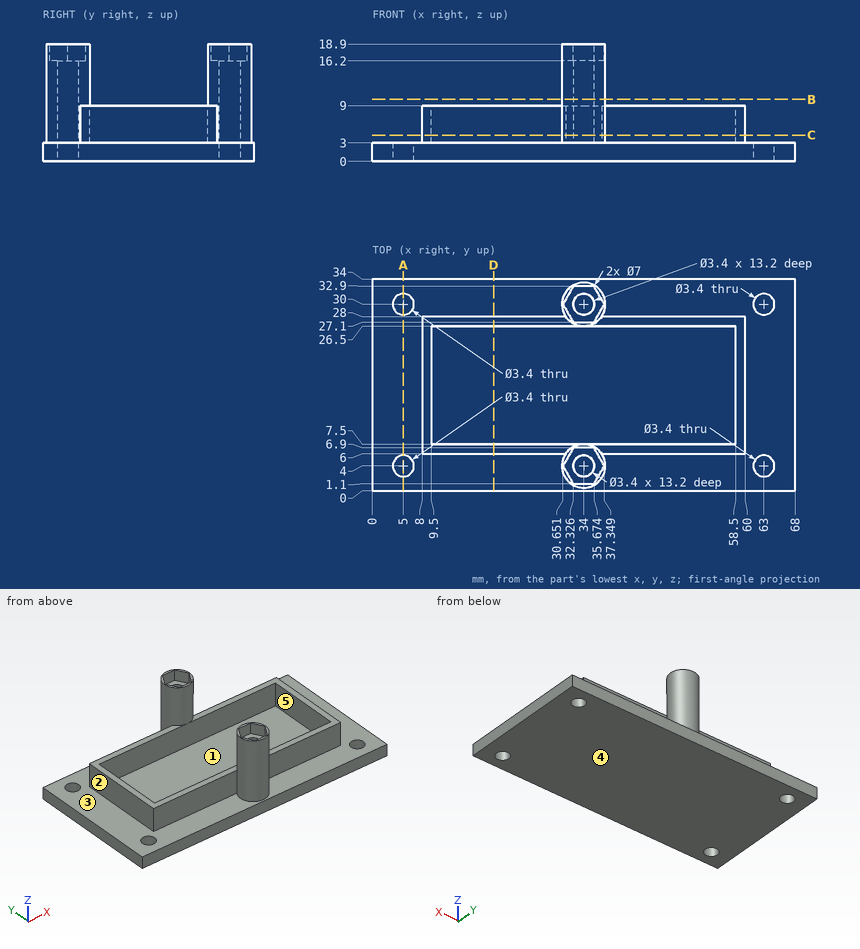
Source: three-view drawing plus pictorial views. Frame: mm from the lowest corner of the part. A direction names the side the tool comes from. Coordinates: 2 decimals unless noted, no trailing zeros. Write each loop counter-clockwise with the first axis right and the second up, starting at its lowest first coordinate (ties: lowest second). Pieces come first, ordered by that corner, then holes. Notation, with made-up numbers: (36, -3.75) - (54, -3.75) arc R17 cw to (54, 9.25) - close; hole circle Ø4 at (87, -13.5). An arc over 180 degrees is marked (long way). Answer as a JSON object with one key per item and string values.
Q1. Set-up query: the marked faces 4 and 5. Return all of +Z, -Z, +X, -X, +Y, -Y with unobstructed straight access to the full face (end or side cutting, diameter ignored); none if empty.
Ans:
{"face 4": "-Z, +X, -X, +Y, -Y", "face 5": "+Z"}
Q2. Section query D-D, the plane x = 19.5. Output: boundary loops of the cut face in (y, z), plus the area to 3 significant figures.
Ans:
{"outline": "(0, 0) - (34, 0) - (34, 3) - (28, 3) - (28, 9) - (26.5, 9) - (26.5, 3) - (7.5, 3) - (7.5, 9) - (6, 9) - (6, 3) - (0, 3) - close", "area": "120 mm2"}
Q3. Draft query along X for the marked faces 1, 2 and 3. Return one class per face: released by +X, released by -X, zero draft, split by the parting line, or undercut.
Ans:
{"face 1": "undercut", "face 2": "released by -X", "face 3": "zero draft"}
Q4. Section query A-A, the plane x = 5. Output: boundary loops of the cut face in (y, z).
Ans:
{"outline": "(0, 0) - (2.3, 0) - (2.3, 3) - (0, 3) - close; (5.7, 0) - (28.3, 0) - (28.3, 3) - (5.7, 3) - close; (31.7, 0) - (34, 0) - (34, 3) - (31.7, 3) - close"}
Q5. Material intervals for line 1 (Y direction, x = 63, z = 2.2); line 2 (Y direction, x = 34, z = 8.75); line 3 (X direction, y = 4, z = 10.5), sorted ascending. Write a range as [from, to].
Ans:
{"line 1": "y = [0, 2.3], [5.7, 28.3], [31.7, 34]", "line 2": "y = [0.5, 2.3], [5.7, 7.5], [26.5, 28.3], [31.7, 33.5]", "line 3": "x = [30.5, 32.3], [35.7, 37.5]"}
Q6. Section query B-B, the plane z = 10. Output: boundary loops of the cut face in (x, y).
Ans:
{"outline": "circle Ø7 at (34, 4); circle Ø7 at (34, 30); hole circle Ø3.4 at (34, 4); hole circle Ø3.4 at (34, 30)"}
Q7. Section query C-C, the plane z = 4.25. Output: boundary loops of the cut face in (x, y).
Ans:
{"outline": "(8, 6) - (31.13, 6) arc R3.5 ccw (long way) to (36.87, 6) - (60, 6) - (60, 28) - (36.87, 28) arc R3.5 ccw (long way) to (31.13, 28) - (8, 28) - close; hole (9.5, 7.5) - (58.5, 7.5) - (58.5, 26.5) - (9.5, 26.5) - close; hole circle Ø3.4 at (34, 4); hole circle Ø3.4 at (34, 30)"}
Q8. First-contact query: pin 1 Ø1.3 at (x, z) = (34, 18) entering from -Y; pin 2 Ø11 at (x, y) = (21, 14.5) entering from +Z; pin 3 Ø0.8 at (x, z) = (33.5, 17.5) entering from +Y; pin 4 Ø2 at (x, y) = (63, 30) entering from +Z. Flat tips, straight axial feed; report the tip coordinate or a pass-through.
Ans:
{"pin 1": "stops at y = 0.5", "pin 2": "stops at z = 3", "pin 3": "stops at y = 33.5", "pin 4": "passes through"}
